Design review of the part built by this model. Coordinates are the model's own, in mm. A direction names the side the tool comes from. Coordinates: 2 decimals unless noted, no trailing zeros. Write each loop counter-clockwise with the first axis right and the second up, starting at its lowest first coordinate (ties: lowest second). Pieces come first, ordered by that corner, then holes. Notation, with made-up numbers: M 73,89 L 113,89 A35 ccw 113,121 Z; hole C 29.25,-36.75 d9. An arc over 180 degrees is marked long. Write each question's results on one line, items separated by ' | '. Start each with the question number.
```python
from build123d import *

# Parameters (mm, degrees)
F0_W     = 21.844
F0_H     = 13.462
F1_DEPTH = 10.414
F2_W     = 14.2748
F2_H     = 13.462
F3_DEPTH = 12.954
F4_R     = 2.3749
F5_DEPTH = 4.826
F7_D     = 2.2606
F7_DEPTH = 9.017
F7_TIP   = 0.6791527577
F9_DEPTH = 13.463


with BuildPart() as f1:
    # F0 (on Front) → F1 (new body)
    with BuildSketch(Plane.XZ):
        Rectangle(F0_W, F0_H)
    extrude(amount=F1_DEPTH)

    # F2 (on face) → F3 (join)
    with BuildSketch(Plane.XZ.offset(10.414)):
        Rectangle(F2_W, F2_H)
    extrude(amount=F3_DEPTH)

    # F4 (on face) → F5 (cut)
    with BuildSketch(Plane.XZ.offset(23.368)):
        Circle(F4_R)
    extrude(amount=-F5_DEPTH, mode=Mode.SUBTRACT)

    # F7
    with Locations(Plane(origin=(0, 0, 0), x_dir=(-1, 0, 0), z_dir=(0, 1, 0))):
        with Locations((7.1374, 0), (-7.1374, 0)):
            Hole(F7_D / 2, depth=F7_DEPTH)
            with Locations((0, 0, -(F7_DEPTH + F7_TIP / 2))):  # 118° drill point
                Cone(0, F7_D / 2, F7_TIP, mode=Mode.SUBTRACT)

    # F8 (on face) → F9 (cut, through all)
    with BuildSketch(Plane.XY.offset(6.731)):
        with BuildLine():
            ThreePointArc((-4.7625, 0), (0, -4.7625), (4.7625, 0))
            Line((4.7625, 0), (-4.7625, 0))
        make_face()
    extrude(amount=-F9_DEPTH, mode=Mode.SUBTRACT)


solid = f1.part
```
Item 1: For faces 4 (the flat face through (8.5, 0, 0.1)), 5 (the flat face through (-9, -10.414, 0)), 6 (the flat face through (0, -18.542, 0)), 7 (the flat face through (9, -10.414, 0)), 8 (the cylindrical face through (8.182, -4.572, -0.433)), list the 3-axis set-ups (+Z, -Z, +X, -X, +Y, -Y) from which the entire face can be reached by the end or side of a thin tool; tool diameter is ignored.
Item 2: We need section B-B on x = 0. State the section outline as (y, z) points.
Item 3: We need section D-D on y = -12. State the section outline as (x, z) points, then the cut area to 3 significant figures.
Item 4: We need section C-C on z = -4.75. State the section outline as (x, y) points (1 decimal), then the cut area to 3 significant figures.
Item 5: Draft analysis for pull direction Z (two halves, no side actions). For faces 1 (the flat face through (0, -12, -6.731)), 2 (the flat face through (-10.922, -5, 0)), 3 (the cylindrical face through (-1.75, -20.989, 1.605)), state which applies: released by +Z, released by -Z, zero draft, split by the parting line, or undercut.
Item 6: Wall thickness on L1, parallel to X at y = -7, z = 0; L2, parallel to X at y = -2, z = 0; L3, parallel to Z at x = 0, y = -21.65: over which ranges is each line inside the solid? List them lowest first.
Item 7: We need section A-A on y = -6.25. State the section outline as (x, z) points.
Item 8: Insertion check: pin 1 Ø5 at (y, z) = (-18.5, -3.5) entering from +X; pin 2 Ø1.9 at (x, z) = (-9, -3) entering from -Y; pin 3 Ø1.4 at (x, z) = (-0.5, -1) entering from -Y. Each pin has a flat end and moves straight along its axis. Give the tip position at first contact, or say it passes through.
Answer:
1) face 4: +Z, -Z, +X, -X, +Y | face 5: +Z, -Z, -X, -Y | face 6: -Y | face 7: +Z, -Z, +X, -Y | face 8: +Y
2) outline: M -23.37,-6.73 L -4.76,-6.73 L -4.76,6.73 L -23.37,6.73 L -23.37,2.37 L -18.54,2.37 L -18.54,-2.37 L -23.37,-2.37 Z
3) outline: M -7.14,-6.73 L 7.14,-6.73 L 7.14,6.73 L -7.14,6.73 Z | area: 192 mm^2
4) outline: M -10.9,-10.4 L -7.1,-10.4 L -7.1,-23.4 L 7.1,-23.4 L 7.1,-10.4 L 10.9,-10.4 L 10.9,0 L 4.8,0 A4.8 cw -4.8,0 L -10.9,0 Z | area: 377 mm^2
5) face 1: released by -Z | face 2: zero draft | face 3: undercut
6) L1: x = -10.92 to -8.27, -6.01 to 6.01, 8.27 to 10.92 | L2: x = -10.92 to -8.27, -6.01 to -4.32, 4.32 to 6.01, 8.27 to 10.92 | L3: z = -6.73 to -2.37, 2.37 to 6.73
7) outline: M -10.92,-6.73 L 10.92,-6.73 L 10.92,6.73 L -10.92,6.73 Z; hole C -7.14,0 d2.26; hole C 7.14,0 d2.26
8) pin 1: stops at x = 7.14 | pin 2: stops at y = -10.41 | pin 3: stops at y = -18.54
